The drawing under review shows one solid part. Ordinate dimensions are in mm from its lowest x, y, z. A direction names the side the tool comes from. Coordinates: 2 decimals unless noted, no trailing zeros. Write each loop counter-clockwise with the first axis right and the second up, starting at its lowest first coordinate (ties: lowest second). Pieces come first, ordered by that corner, then holes.
Q1. Take a section at C-C (z = 20). Give the boundary of the cut face in (x, y) (3 decimals).
Q2. Machinability: for the marked faces 5 and 6, which of the approach directions +Z, -Z, +X, -X, +Y, -Y give a long, thin tool a straight path to every point of the face, cutting with its end or side? Answer none if there is none.
Q3. Take a section at D-D (x = 35). Give the boundary of the cut face in (y, z) (3 decimals).
Q4. For probe 1 along Z at (x, y) = (19, 13) (3 decimals); probe 2 along Y at (x, z) = (30.5, 8) (3 decimals), list the stretches that pass through material, from the lowest coordinate up.
Q5. Insertion check: pin 1 (3 mm diameter, centred on y = 7.5, z = 2.5, fed in from +X). The pin has a flat end and moves straight along its axis. Give the tip position at first contact, or say it passes through.
Q6. Take a section at B-B (x = 4.5). Give the boundary of the cut face in (y, z) (3 decimals), and give its area (3 significant figures).
Q7. Mouldability with a two-part tool opening along Y and no side actions: class the marked faces 1, 2, 3 and 4 as pulls with the +Y half, pulls with the -Y half, needs draft (parallel to the pull), parting line crosses it, or undercut.
Q8. Take a section at A-A (y = 15.5). Give the boundary of the cut face in (x, z) (3 decimals), and give its area (3 significant figures).
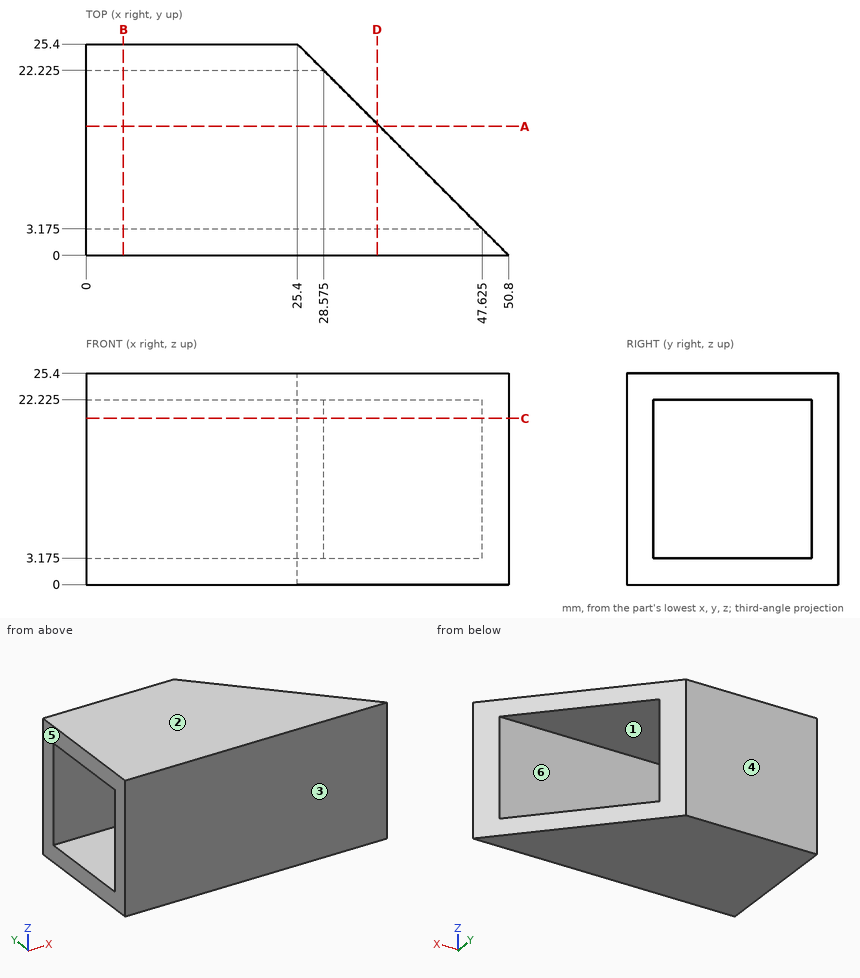
Response:
1. outline: (0, 0) - (50.8, 0) - (47.625, 3.175) - (0, 3.175) - close; (0, 22.225) - (28.575, 22.225) - (25.4, 25.4) - (0, 25.4) - close
2. face 5: +Z, -Z, -X, +Y, -Y
2. face 6: +X, -X
3. outline: (0, 0) - (15.8, 0) - (15.8, 3.175) - (3.175, 3.175) - (3.175, 22.225) - (15.8, 22.225) - (15.8, 25.4) - (0, 25.4) - close
4. probe 1: z = 0 to 3.175, 22.225 to 25.4
4. probe 2: y = 0 to 3.175
5. pin 1: stops at x = 44.8
6. outline: (0, 0) - (25.4, 0) - (25.4, 25.4) - (0, 25.4) - close; hole (3.175, 3.175) - (22.225, 3.175) - (22.225, 22.225) - (3.175, 22.225) - close
6. area: 282 mm2
7. face 1: undercut
7. face 2: needs draft
7. face 3: pulls with the -Y half
7. face 4: pulls with the +Y half
8. outline: (0, 0) - (35.3, 0) - (35.3, 3.175) - (0, 3.175) - close; (0, 22.225) - (35.3, 22.225) - (35.3, 25.4) - (0, 25.4) - close
8. area: 224 mm2
